from build123d import *

# Parameters (mm, degrees)
SKETCH1_R                = 63.66
BOSS_EXTRUDE1_DEPTH      = 10
SKETCH2_R                = 65
BOSS_EXTRUDE2_DEPTH      = 2
BOSS_EXTRUDE3_DEPTH      = 10
BOSS_EXTRUDE3_DEPTH_BACK = 2
SKETCH3_R                = 65
SKETCH4_R                = 2.5
SKETCH4_R_2              = 44
CUT_EXTRUDE1_DEPTH       = 95.074438611
SKETCH5_R                = 50
CUT_EXTRUDE2_DEPTH       = 10


with BuildPart() as part:
    # Sketch1 → Boss-Extrude1 (new body)
    with BuildSketch(Plane(origin=(0, 0, 0), x_dir=(1, 0, 0), z_dir=(0, 1, 0))):
        with Locations(Location((0, 0, 0), (0, 0, 270))):
            Circle(SKETCH1_R)
    extrude(amount=BOSS_EXTRUDE1_DEPTH)

    # Sketch2 → Boss-Extrude2 (add)
    with BuildSketch(Plane(origin=(0, 10, 0), x_dir=(1, 0, 0), z_dir=(0, 1, 0))):
        with Locations(Location((0, 0, 0), (0, 0, 270))):
            Circle(SKETCH2_R)
    extrude(amount=-BOSS_EXTRUDE2_DEPTH)

    # Sketch3 → Boss-Extrude3 (add, two sides: drawn at the far end of the back side and taken through both)
    with BuildSketch(Plane.XZ.offset(-BOSS_EXTRUDE3_DEPTH_BACK)):
        with Locations(Location((0, 0, 0), (0, 0, 90))):
            Circle(SKETCH3_R)
    extrude(amount=BOSS_EXTRUDE3_DEPTH + BOSS_EXTRUDE3_DEPTH_BACK)

    # Sketch4 → Cut-Extrude1 (cut, through all)
    with BuildSketch(Plane(origin=(0, 10, 0), x_dir=(1, 0, 0), z_dir=(0, 1, 0))):
        with Locations(Location((0, 56.5, 0), (0, 0, 270))):
            Circle(SKETCH4_R)
        with Locations(Location((39.951533137, 39.951533137, 0), (0, 0, 270))):
            Circle(SKETCH4_R)
        with Locations(Location((56.5, 0, 0), (0, 0, 270))):
            Circle(SKETCH4_R)
        with Locations(Location((39.951533137, -39.951533137, 0), (0, 0, 270))):
            Circle(SKETCH4_R)
        with Locations(Location((0, -56.5, 0), (0, 0, 270))):
            Circle(SKETCH4_R)
        with Locations(Location((-39.951533137, -39.951533137, 0), (0, 0, 270))):
            Circle(SKETCH4_R)
        with Locations(Location((-56.5, 0, 0), (0, 0, 270))):
            Circle(SKETCH4_R)
        with Locations(Location((-39.951533137, 39.951533137, 0), (0, 0, 270))):
            Circle(SKETCH4_R)
        with Locations(Location((0, 0, 0), (0, 0, 270))):
            Circle(SKETCH4_R_2)
    extrude(amount=-CUT_EXTRUDE1_DEPTH, mode=Mode.SUBTRACT)

    # Sketch5 → Cut-Extrude2 (cut)
    with BuildSketch(Plane(origin=(0, 10, 0), x_dir=(1, 0, 0), z_dir=(0, 1, 0))):
        with Locations(Location((0, 0, 0), (0, 0, 270))):
            Circle(SKETCH5_R)
    extrude(amount=-CUT_EXTRUDE2_DEPTH, mode=Mode.SUBTRACT)


solid = part.part
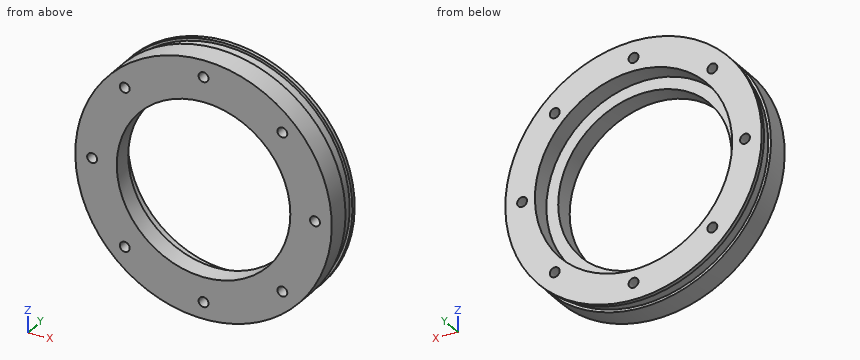
Model file for the job. Use its own axes, mm. Give positions to 0.01 mm unless a question says otherwise; leave off trailing zeros. Loops run counter-clockwise (first coordinate to the right, second up) from the corner with the lowest first, then second, coordinate; pieces in that order, holes last.
1) Saw through at B-B (z = -40.5). Write the cut outline in (x, y).
2) Saw through at A-A (x = 0). Write the cut outline in (y, z).
3) Flat gauge pins, fed straight in: pin 1 Ø5 at (x, y) = (43, 5.5) entering from +Z; pin 2 Ø4 at (y, z) = (-0.5, 24.5) entering from +X; pin 3 Ø6 at (x, z) = (-56.5, 0) entering from +Y; pin 4 Ø5 at (x, y) = (-27, 6) entering from -Z. Where does each tip first touch, or does it go through?
4) Wall check: line 1 (X direction, y = 3.5, z = 0); line 2 (X direction, y = -2.5, z = 0); line 3 (Z direction, x = 40, y = -6). Give the ranges that are in metal, low to high.
5) Saw through at C-C (z = 56.5). Write the cut outline in (x, y), plus the area to 3 significant figures.
6) Saw through at D-D (x = -56.5). Write the cut outline in (y, z).
Answer block:
1. outline: (-50.84, -10) - (-42.39, -10) - (-42.39, 10) - (-50.84, 10) - (-50.84, 8) - (-49.12, 8) - (-49.12, 2) - (-50.84, 2) - close; (-37.51, -10) - (-17.2, -10) - (-17.2, 0) - (-29.32, 0) - (-29.32, 10) - (-37.51, 10) - close; (17.2, -10) - (37.51, -10) - (37.51, 10) - (29.32, 10) - (29.32, 0) - (17.2, 0) - close; (42.39, -10) - (50.84, -10) - (50.84, 2) - (49.12, 2) - (49.12, 8) - (50.84, 8) - (50.84, 10) - (42.39, 10) - close
2. outline: (-10, -65) - (2, -65) - (2, -63.66) - (8, -63.66) - (8, -65) - (10, -65) - (10, -59) - (-10, -59) - close; (-10, -54) - (10, -54) - (10, -50) - (0, -50) - (0, -44) - (-10, -44) - close; (-10, 44) - (0, 44) - (0, 50) - (10, 50) - (10, 54) - (-10, 54) - close; (-10, 59) - (10, 59) - (10, 65) - (8, 65) - (8, 63.66) - (2, 63.66) - (2, 65) - (-10, 65) - close
3. pin 1: stops at z = 49.12
3. pin 2: stops at x = 60.98
3. pin 3: stops at y = 10
3. pin 4: stops at z = -59.79
4. line 1: x = -63.66 to -59, -54 to -50, 50 to 54, 59 to 63.66
4. line 2: x = -65 to -59, -54 to -44, 44 to 54, 59 to 65
4. line 3: z = -51.23 to -42.45, -37.45 to -18.33, 18.33 to 37.45, 42.45 to 51.23
5. outline: (-32.14, -10) - (-2.5, -10) - (-2.5, 10) - (-32.14, 10) - (-32.14, 8) - (-29.33, 8) - (-29.33, 2) - (-32.14, 2) - close; (2.5, -10) - (32.14, -10) - (32.14, 2) - (29.33, 2) - (29.33, 8) - (32.14, 8) - (32.14, 10) - (2.5, 10) - close
5. area: 1,150 mm2
6. outline: (-10, -32.14) - (2, -32.14) - (2, -29.33) - (8, -29.33) - (8, -32.14) - (10, -32.14) - (10, -2.5) - (-10, -2.5) - close; (-10, 2.5) - (10, 2.5) - (10, 32.14) - (8, 32.14) - (8, 29.33) - (2, 29.33) - (2, 32.14) - (-10, 32.14) - close
